Source: CAD feature listing. Evaluate the final solid. Frame: model axes, mm. Face numbers are marked on the shaded views. A direction names the side the tool comes from. Give positions to 0.01 mm unless a question says otherwise; leave off trailing zeros. Order: outer loops, then holes, each group sorted by start corner. A loop starts at its lowest first (then second) coordinate and runs counter-clockwise, first axis right, second up.
from build123d import *

# Parameters (mm, degrees)
EXTRUDE_START       = -4
EXTRUDE_1_DEPTH     = 8
SKETCH_2_R          = 3
SKETCH_2_R_2        = 1.5
CUT_EXTRUDE_1_DEPTH = 135.118611684


with BuildPart() as part:
    # 草图1 → 凸台-拉伸1 (new body)
    with BuildSketch(Plane(origin=(0, 0, 0), x_dir=(1, 0, 0), z_dir=(0, 1, 0)).offset(EXTRUDE_START)):
        Polygon((104.32, -54.86), (122.32, -38.86), (113.32, -28.735), (95.32, -44.735), align=None)
    extrude(amount=EXTRUDE_1_DEPTH)

    # 草图2 → 切除-拉伸1 (cut, through all)
    with BuildSketch(Plane(origin=(0, 0, 0), x_dir=(1, 0, 0), z_dir=(0, 1, 0))):
        with Locations((100, -50)):
            Circle(SKETCH_2_R)
        with Locations(Location((114, -38, 0), (0, 0, 270))):
            Circle(SKETCH_2_R_2)
    extrude(amount=-CUT_EXTRUDE_1_DEPTH, mode=Mode.SUBTRACT)


solid = part.part
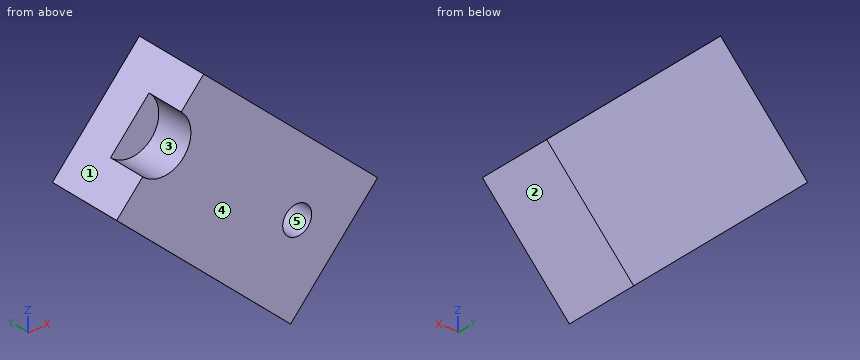
1) Section query C-C on x = 100. Output: boundary loops of the cut face in (y, z) (3 decimals).
Checks:
outline: (-4, 40.575) - (4, 40.575) - (4, 50) - (0, 50) - (0, 47) - (-4, 47) - close
2) Pull-direction query (Z, two-part tool) for the marked faces 1, 2 and 3; classes: +Z half, -Z half, draft (parallel to the pull), parting line (faces both ways), or undercut.
Checks:
face 1: +Z half
face 2: -Z half
face 3: undercut
3) Ray query, L1, parallel to Z at x = 114, y = -2.15; L2, parallel to X at y = -0.95, z = 38; L3, parallel to Z at x = 111.5, y = 3. Return the intervals inside material, ascending.
Checks:
L1: z = 29.5 to 36.5, 39.5 to 46.26
L2: x = 102.9 to 112.5, 115.5 to 121.56
L3: z = 30.35 to 48.48
4) Section query D-D on y = 3. Output: boundary loops of the cut face in (x, z) (3 decimals).
Checks:
outline: (95.32, 44.735) - (113.32, 28.735) - (122.32, 38.86) - (104.32, 54.86) - close
5) Section query B-B on z = 38. Output: boundary loops of the cut face in (x, y).
Checks:
outline: (102.9, -4) - (112.5, -4) - (112.5, 0) - (115.5, 0) - (115.5, -4) - (121.56, -4) - (121.56, 4) - (102.9, 4) - close
6) Reachability of the marked faces 4 and 5 from +Z, -Z, +X, -X, +Y, -Y: full face, straight path, thin tool, end or side. Return the list, or none.
Checks:
face 4: +Z, -Z, +X, -X, -Y
face 5: -Y
7) First-contact query: pin 1 Ø2 at (y, z) = (2.5, 32) entering from -X; pin 2 Ø4 at (x, y) = (104, -0.5) entering from -Z; pin 3 Ø2.5 at (x, z) = (100, 51) entering from -Y. Flat tips, straight axial feed; report the tip coordinate or a pass-through.
Checks:
pin 1: stops at x = 108.52
pin 2: stops at z = 35.24
pin 3: stops at y = 0
8) Section query A-A on y = -2.25. Output: boundary loops of the cut face in (x, z) (3 decimals), and give its area (3 significant figures).
Checks:
outline: (95.32, 44.735) - (113.32, 28.735) - (122.32, 38.86) - (104.32, 54.86) - (101.993, 52.242) arc R3 cw to (98.007, 47.758) - close; hole circle Ø3 at (114, 38)
area: 305 mm2
